```python
from build123d import *

# Parameters (mm, degrees)
SKETCH1_R                            = 2.0193
BOSS_EXTRUDE1_DEPTH                  = 331.7875
SKETCH2_R                            = 8.89
SKETCH2_R_2                          = 6.35
CUT_EXTRUDE_THIN1_DEPTH              = 7.9375
SKETCH3_W                            = 2.21098701
SKETCH3_H                            = 0.9906
SKETCH3_W_2                          = 2.67360648
F_10_32_TAPPED_HOLE1_D               = 4.0386
F_10_32_TAPPED_HOLE1_DEPTH           = 12.02944
F_10_32_TAPPED_HOLE1_TIP             = 1.213317848
F_10_32_TAPPED_HOLE1_ON_FACE_2_D     = 4.0386
F_10_32_TAPPED_HOLE1_ON_FACE_2_DEPTH = 12.02944
F_10_32_TAPPED_HOLE1_ON_FACE_2_TIP   = 1.213317848


with BuildPart() as part:
    # Sketch1 → Boss-Extrude1 (new, symmetric)
    with BuildSketch(Plane.XY):
        with BuildLine():
            ThreePointArc((0.893039571, 6.816751782), (0, 6.874999966), (-0.893039571, 6.816751782))
            Line((-0.893039571, 6.816751782), (-5.456960429, 4.181770846))
            ThreePointArc((-5.456960429, 4.181770846), (-5.953924622, 3.437499983), (-6.35, 2.634980936))
            Line((-6.35, 2.634980936), (-6.35, -2.634980936))
            ThreePointArc((-6.35, -2.634980936), (-5.953924622, -3.437499983), (-5.456960429, -4.181770846))
            Line((-5.456960429, -4.181770846), (-0.893039571, -6.816751782))
            ThreePointArc((-0.893039571, -6.816751782), (0, -6.874999966), (0.893039571, -6.816751782))
            Line((0.893039571, -6.816751782), (5.456960429, -4.181770846))
            ThreePointArc((5.456960429, -4.181770846), (5.953924622, -3.437499983), (6.35, -2.634980936))
            Line((6.35, -2.634980936), (6.35, 2.634980936))
            ThreePointArc((6.35, 2.634980936), (5.953924622, 3.437499983), (5.456960429, 4.181770846))
            Line((5.456960429, 4.181770846), (0.893039571, 6.816751782))
        make_face()
        Circle(SKETCH1_R, mode=Mode.SUBTRACT)
    extrude(amount=BOSS_EXTRUDE1_DEPTH, both=True)

    # Sketch2 → Cut-Extrude-Thin1 (cut)
    with BuildSketch(Plane(origin=(0, 0, -331.7875), x_dir=(-1, 0, 0), z_dir=(0, 0, -1))):
        Circle(SKETCH2_R)
        Circle(SKETCH2_R_2, mode=Mode.SUBTRACT)
    cut_extrude_thin1 = extrude(amount=-CUT_EXTRUDE_THIN1_DEPTH, mode=Mode.SUBTRACT)

    # Sketch3 → Cut-Revolve4 (revolve, cut)
    with BuildSketch(Plane(origin=(0, 0, 0), x_dir=(1, 0, 0), z_dir=(0, 1, 0))):
        with Locations((7.049093505, -290.0172)):
            Rectangle(SKETCH3_W, SKETCH3_H)
        with Locations((7.28040324, 277.3172)):
            Rectangle(SKETCH3_W_2, SKETCH3_H)
    revolve(axis=Axis((0, 0, -323.85), (0, 0, -1)), mode=Mode.SUBTRACT)

    # Mirror1: Cut-Extrude-Thin1 across plane
    add(cut_extrude_thin1.mirror(Plane.XY), mode=Mode.SUBTRACT)

    # #10-32 Tapped Hole1
    with Locations(Plane(origin=(0, 0, -331.7875), x_dir=(-1, 0, 0), z_dir=(0, 0, -1))):
        with Locations((0, 0)):
            Hole(F_10_32_TAPPED_HOLE1_D / 2, depth=F_10_32_TAPPED_HOLE1_DEPTH)
            with Locations((0, 0, -(F_10_32_TAPPED_HOLE1_DEPTH + F_10_32_TAPPED_HOLE1_TIP / 2))):  # 118° drill point
                Cone(0, F_10_32_TAPPED_HOLE1_D / 2, F_10_32_TAPPED_HOLE1_TIP, mode=Mode.SUBTRACT)

    # #10-32 Tapped Hole1 on face 2
    with Locations(Plane(origin=(0, 0, 331.7875), x_dir=(-1, 0, 0), z_dir=(0, 0, -1))):
        with Locations((0, 0)):
            Hole(F_10_32_TAPPED_HOLE1_ON_FACE_2_D / 2, depth=F_10_32_TAPPED_HOLE1_ON_FACE_2_DEPTH)
            with Locations((0, 0, -(F_10_32_TAPPED_HOLE1_ON_FACE_2_DEPTH + F_10_32_TAPPED_HOLE1_ON_FACE_2_TIP / 2))):  # 118° drill point
                Cone(0, F_10_32_TAPPED_HOLE1_ON_FACE_2_D / 2, F_10_32_TAPPED_HOLE1_ON_FACE_2_TIP, mode=Mode.SUBTRACT)


solid = part.part
```
CAD build for the part. Positions are in the model's coordinates, mm. A direction names the side the tool comes from. Coordinates: 2 decimals unless noted, no trailing zeros. Write each loop counter-clockwise with the first axis right and the second up, starting at its lowest first coordinate (ties: lowest second). Pieces come first, ordered by that corner, then holes. Notation, with made-up numbers: (65, -22.5) -> (96, -22.5) arc R26 cw to (96, 3.5) -> close; hole circle Ø9 at (41, 74). An arc over 180 degrees is marked (long way). Use CSV: the item, a comma, the result in double quotes. Start each with the question number.
Item 1: Wall check: probe 1 along Z at (x, y) = (5, 4); probe 2 along Y at (x, z) = (0, 125.5) (3 decimals); probe 3 along X at (y, z) = (0.5, 269). Give the ranges that are in metal, low to high.
Item 2: Tool access for faces 1 (the cylindrical face through (1.38, -6.2, -327.87)), 2 (the flat face through (5, -4, -276.822)), 3 (the cylindrical face through (1.38, -6.2, 327.87)): list every direction of +Z, -Z, +X, -X, +Y, -Y with a clear straight run to the whole face (end or side of a thin tool).
Item 3: Band-saw the part on A-A, the plane z = -139. Write the cut outline in (x, y) (3 decimals), plus the area to 3 significant figures.
Item 4: Drop flat-ended pins along their axis: P1, Ø1.5, axis at x = -2, z = 241.5, coming from the -Y side; P2, Ø1.5, axis at y = 4, z = -50, coming from the +X side; P3, Ø2, axis at x = 1.5, z = 258, coming from the +Y side. Give the stop position or say it passes through.
Response values:
1,probe 1,"z = -323.85 to -277.81, -276.82 to 289.52, 290.51 to 323.85"
1,probe 2,"y = -6.875 to -2.019, 2.019 to 6.875"
1,probe 3,"x = -6.35 to -1.96, 1.96 to 6.35"
2,face 1,"-Z"
2,face 2,"none"
2,face 3,"+Z"
3,outline,"(-6.35, -2.635) arc R6.875 ccw to (-5.457, -4.182) -> (-0.893, -6.817) arc R6.875 ccw to (0.893, -6.817) -> (5.457, -4.182) arc R6.875 ccw to (6.35, -2.635) -> (6.35, 2.635) arc R6.875 ccw to (5.457, 4.182) -> (0.893, 6.817) arc R6.875 ccw to (-0.893, 6.817) -> (-5.457, 4.182) arc R6.875 ccw to (-6.35, 2.635) -> close; hole circle Ø4.039 at (0, 0)"
3,area,"125 mm2"
4,P1,"stops at y = -6.61"
4,P2,"stops at x = 6.06"
4,P3,"stops at y = 6.86"
